Model file for the job. Use its own axes, mm. A direction names the side the tool comes from. Give positions to 0.01 mm unless a question says otherwise; leave off trailing zeros. Write each loop counter-clockwise with the first axis right and the second up, starting at its lowest first coordinate (ties: lowest second). Pieces come first, ordered by that corner, then holes. Notation, with made-up numbers: M 5.5,76 L 40.5,76 A20 ccw 40.5,115 Z; hole C -35,16 d10. An arc over 180 degrees is marked long. Answer as a JSON object with one key per item and string values. Group by question number.
```python
from build123d import *

# Parameters (mm, degrees)
EXTRUDE_THIN1_DEPTH = 81.5
SKETCH2_W           = 37
SKETCH2_H           = 40
CUT_EXTRUDE1_DEPTH  = 10
SKETCH3_R           = 4.1
CUT_EXTRUDE2_DEPTH  = 10
SKETCH4_R           = 3.1
CUT_EXTRUDE3_DEPTH  = 10
FILLET1_R           = 5


with BuildPart() as part:
    # Sketch1 → Extrude-Thin1 (new body)
    with BuildSketch(Plane(origin=(0, 0, 0), x_dir=(1, 0, 0), z_dir=(0, 1, 0))):
        with BuildLine():
            Line((40, 0), (3, 0))
            ThreePointArc((3, 0), (0.878679656, -0.878679656), (0, -3))
            Line((0, -3), (0, -40))
            Line((0, -40), (3, -40))
            Line((3, -40), (3, -3))
            Line((3, -3), (40, -3))
            Line((40, -3), (40, 0))
        make_face()
    extrude(amount=EXTRUDE_THIN1_DEPTH)

    # Sketch2 → Cut-Extrude1 (cut)
    with BuildSketch(Plane(origin=(3, 0, 0), x_dir=(0, 0, -1), z_dir=(1, 0, 0))):
        with Locations((-21.5, 61.5)):
            Rectangle(SKETCH2_W, SKETCH2_H)
    extrude(amount=-CUT_EXTRUDE1_DEPTH, mode=Mode.SUBTRACT)

    # Sketch3 → Cut-Extrude2 (cut)
    with BuildSketch(Plane(origin=(0, 0, 0), x_dir=(-1, 0, 0), z_dir=(0, 0, -1))):
        with Locations((-20, 61.5)):
            Circle(SKETCH3_R)
    extrude(amount=-CUT_EXTRUDE2_DEPTH, mode=Mode.SUBTRACT)

    # Sketch4 → Cut-Extrude3 (cut)
    with BuildSketch(Plane(origin=(0, 0, 0), x_dir=(-1, 0, 0), z_dir=(0, 0, -1))):
        with Locations((-20, 9)):
            Circle(SKETCH4_R)
        with Locations((-20, 34)):
            Circle(SKETCH4_R)
    extrude(amount=-CUT_EXTRUDE3_DEPTH, mode=Mode.SUBTRACT)

    # Fillet1
    fillet1_edges = [part.edges().sort_by_distance(p)[0] for p in [
        (1.5, 41.5, 40),
        (1.5, 0, 40),
        (40, 81.5, 1.5),
        (40, 0, 1.5),
    ]]
    fillet(fillet1_edges, radius=FILLET1_R)


solid = part.part
```
Q1. Slice it at A-A, the plane x = 20. Write the cut outline in (y, z).
Q2. Wall check: L1, parallel to Y at x = 20, z = 0.8; L2, parallel to X at y = 22.5, z = 31.5. Give the ranges that are in metal, low to high.
Q3. Slice it at D-D, the plane y = 9. Write the cut outline in (x, z).
Q4. Two-plate mould, pull along Y, no slides. Class faces 3 (the flat face through (2, 0, 10)), 4 (the cylindrical face through (23.022, 64.271, 1.479)), 5 (the flat face through (3, 20, 22)): +Y half, -Y half, draft (parallel to the pull), parting line (faces both ways), or undercut.
Q5. Slice it at C-C, the plane y = 40.5. Write the cut outline in (x, z).
Q6. 3-axis set-ups, long thin cutter, end or side, ignore diameter. For faces 1 (the flat face through (1, 21, 40)), 2 (the flat face through (2, 41.5, 19)): which of +Z, -Z, +X, -X, +Y, -Y reach the whole face in a straight line?
Q7. Slice it at B-B, the plane y = 61.5. Write the cut outline in (x, z), then the cut area to 3 significant figures.
Q8. Drop flat-ended pins along their axis: P1, Ø2, axis at x = 19.5, y = 33, coming from the -Z side; P2, Ø0.9, axis at x = 1.5, z = 19, coming from the +Y side; P3, Ø2, axis at x = 32.5, y = 40.5, coming from the +Z side. Give the stop position or say it passes through.
Solved:
{
 "1": {"outline": "M 0,0 L 5.9,0 L 5.9,3 L 0,3 Z; M 12.1,0 L 30.9,0 L 30.9,3 L 12.1,3 Z; M 37.1,0 L 57.4,0 L 57.4,3 L 37.1,3 Z; M 65.6,0 L 81.5,0 L 81.5,3 L 65.6,3 Z"},
 "2": {"L1": "y = 0 to 5.9, 12.1 to 30.9, 37.1 to 57.4, 65.6 to 81.5", "L2": "x = 0 to 3"},
 "3": {"outline": "M 0,3 A3 ccw 3,0 L 16.9,0 L 16.9,3 L 3,3 L 3,40 L 0,40 Z; M 23.1,0 L 40,0 L 40,3 L 23.1,3 Z"},
 "4": {"face 3": "-Y half", "face 4": "undercut", "face 5": "draft"},
 "5": {"outline": "M 0,3 A3 ccw 3,0 L 40,0 L 40,3 L 3,3 L 3,38 L 0,38 Z"},
 "6": {"face 1": "+Z, +X, -X, +Y, -Y", "face 2": "+Z, +X, -X, +Y"},
 "7": {"outline": "M 0,3 A3 ccw 3,0 L 15.9,0 L 15.9,3 Z; M 24.1,0 L 40,0 L 40,3 L 24.1,3 Z", "area": "93.5 mm²"},
 "8": {"P1": "passes through", "P2": "stops at y = 41.5", "P3": "stops at z = 3"}
}
